Could you check a few things on this model? Use its own coordinates, in mm. Face numbers are marked on the shaded views. A direction names the side the tool comes from. Round coordinates to 2 decimals unless told otherwise and drop trailing zeros. Loops run counter-clockwise (first coordinate to the right, second up) from the corner with the lowest first, then second, coordinate; pieces in that order, holes last. Notation, with made-up numbers: (84, 44.25) -> (98, 44.25) arc R20 cw to (98, 81.25) -> close; hole circle Ø4 at (21, 40). An arc over 180 degrees is marked (long way). Write each question's results on one line, items separated by ' | '.
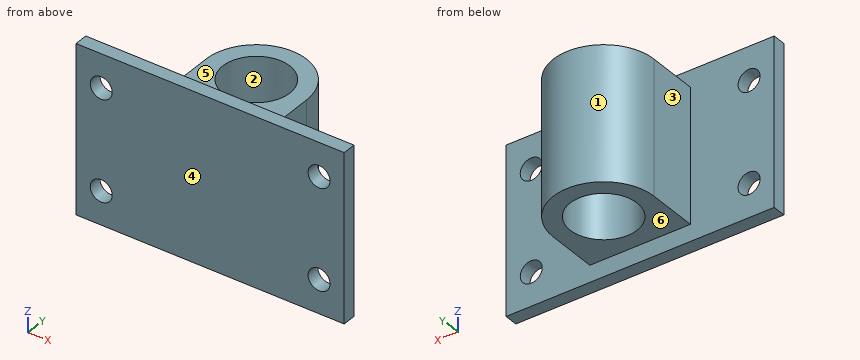
from build123d import *

# Parameters (mm, degrees)
SKETCH1_W           = 101.6
SKETCH1_H           = 63.5
BOSS_EXTRUDE1_DEPTH = 5.08
SKETCH2_R           = 4.1656
CUT_EXTRUDE1_DEPTH  = 61.120785923
SKETCH3_R           = 12.7
BOSS_EXTRUDE2_DEPTH = 25.4


with BuildPart() as part:
    # Sketch1 → Boss-Extrude1 (new body)
    with BuildSketch(Plane(origin=(0, 0, 0), x_dir=(1, 0, 0), z_dir=(0, 1, 0))):
        Rectangle(SKETCH1_W, SKETCH1_H)
    extrude(amount=BOSS_EXTRUDE1_DEPTH)

    # Sketch2 → Cut-Extrude1 (cut, through all)
    with BuildSketch(Plane(origin=(0, 0, 0), x_dir=(1, 0, 0), z_dir=(0, 1, 0))):
        with Locations(Location((-41.275, 19.05, 0), (0, 0, 270))):
            Circle(SKETCH2_R)
        with Locations(Location((41.275, 19.05, 0), (0, 0, 270))):
            Circle(SKETCH2_R)
        with Locations(Location((41.275, -19.05, 0), (0, 0, 270))):
            Circle(SKETCH2_R)
        with Locations(Location((-41.275, -19.05, 0), (0, 0, 270))):
            Circle(SKETCH2_R)
    extrude(amount=CUT_EXTRUDE1_DEPTH, mode=Mode.SUBTRACT)

    # Sketch3 → Boss-Extrude2 (add, symmetric)
    with BuildSketch(Plane.XY):
        with BuildLine():
            Line((-19.05, 24.13), (-19.05, 5.08))
            Line((-19.05, 5.08), (19.05, 5.08))
            Line((19.05, 5.08), (19.05, 24.13))
            ThreePointArc((19.05, 24.13), (0, 43.18), (-19.05, 24.13))
        make_face()
        with Locations((0, 24.13)):
            Circle(SKETCH3_R, mode=Mode.SUBTRACT)
    extrude(amount=BOSS_EXTRUDE2_DEPTH, both=True)


solid = part.part
1) I'm going to push flat-ended pins straight in: pin 1 (1 mm diameter, centred on y = 28.5, z = -3, fed in from +X); pin 2 (10 mm diameter, centred on x = 23, y = 19, fed in from -Z); pin 3 (5 mm diameter, centred on y = 12.5, z = 21.5, fed in from +X). Where does each tip first touch, or does it pass through?
Model answer:
pin 1: stops at x = 18.65 | pin 2: stops at z = -25.4 | pin 3: stops at x = 19.05
2) For the marked faces 4, 5 and 6, which set-ups out of +Z, -Z, +X, -X, +Y, -Y let a thin tool reach every point of the face, with its end or its side?
Model answer:
face 4: +Z, -Z, +X, -X, -Y | face 5: +Z, +X, -X, +Y | face 6: -Z, +X, -X, +Y
3) I want a section at A-A, the plane x = 0. Write out the boundary of the cut face in (y, z).
Model answer:
outline: (0, -31.75) -> (5.08, -31.75) -> (5.08, -25.4) -> (11.43, -25.4) -> (11.43, 25.4) -> (5.08, 25.4) -> (5.08, 31.75) -> (0, 31.75) -> close; (36.83, -25.4) -> (43.18, -25.4) -> (43.18, 25.4) -> (36.83, 25.4) -> close
4) I need wall thicknesses on line 1 (X direction, y = 3.4, z = -19.05); line 2 (Y direction, x = 0.5, z = -10.5); line 3 (X direction, y = 2.5, z = -21). Which ranges of each line are inside material? Lowest first, please.
Model answer:
line 1: x = -50.8 to -45.44, -37.11 to 37.11, 45.44 to 50.8 | line 2: y = 0 to 11.44, 36.82 to 43.17 | line 3: x = -50.8 to -44.96, -37.59 to 37.59, 44.96 to 50.8
5) I want a section at B-B, the plane z = -19.05. Write out the boundary of the cut face in (x, y).
Model answer:
outline: (-50.8, 0) -> (-45.44, 0) -> (-45.44, 5.08) -> (-50.8, 5.08) -> close; (-37.11, 0) -> (37.11, 0) -> (37.11, 5.08) -> (19.05, 5.08) -> (19.05, 24.13) arc R19.05 ccw to (-19.05, 24.13) -> (-19.05, 5.08) -> (-37.11, 5.08) -> close; (45.44, 0) -> (50.8, 0) -> (50.8, 5.08) -> (45.44, 5.08) -> close; hole circle Ø25.4 at (0, 24.13)
6) If we mould it in two halves opening along Y, with no side actions, what happens to the marked faces 1, 2 and 3? For each: released by +Y, released by -Y, zero draft, split by the parting line, or undercut.
Model answer:
face 1: released by +Y | face 2: undercut | face 3: zero draft
7) I want a section at D-D, the plane x = 39. Write out the boundary of the cut face in (y, z), plus the area to 3 significant figures.
Model answer:
outline: (0, -31.75) -> (5.08, -31.75) -> (5.08, -22.54) -> (0, -22.54) -> close; (0, -15.56) -> (5.08, -15.56) -> (5.08, 15.56) -> (0, 15.56) -> close; (0, 22.54) -> (5.08, 22.54) -> (5.08, 31.75) -> (0, 31.75) -> close | area: 252 mm2
8) I want a section at C-C, the plane z = 10.5. Write out the boundary of the cut face in (x, y).
Model answer:
outline: (-50.8, 0) -> (50.8, 0) -> (50.8, 5.08) -> (19.05, 5.08) -> (19.05, 24.13) arc R19.05 ccw to (-19.05, 24.13) -> (-19.05, 5.08) -> (-50.8, 5.08) -> close; hole circle Ø25.4 at (0, 24.13)
